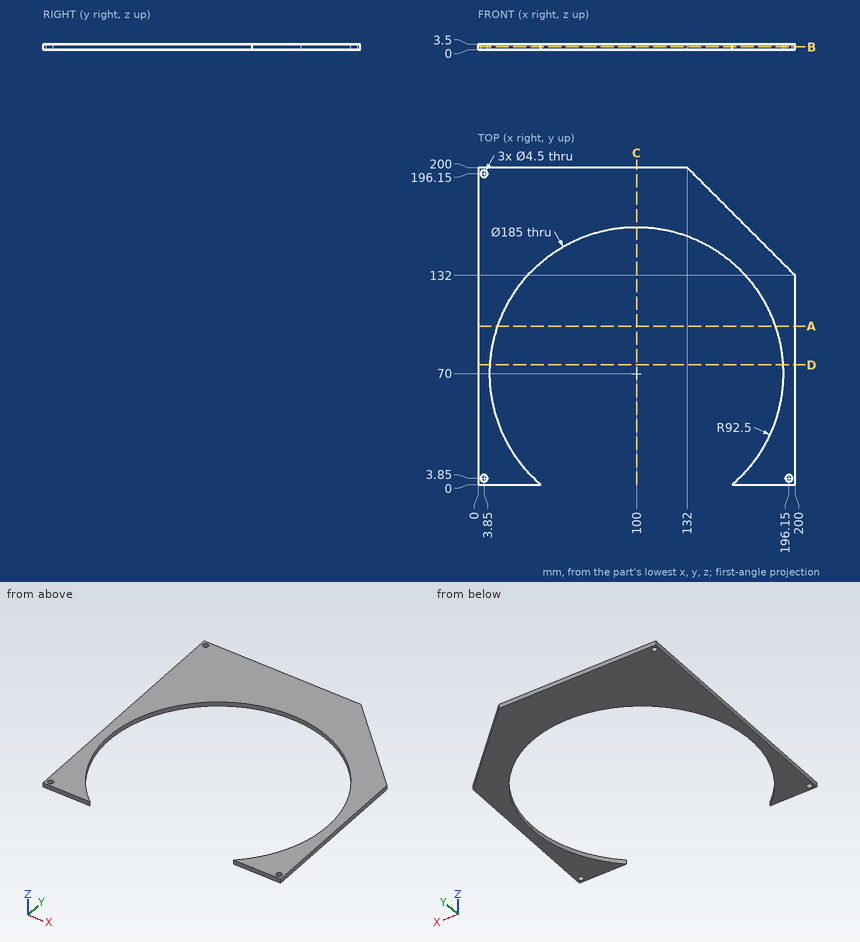
Job drawing, mm, ordinate dimensions from the low corner. One solid piece. Coordinates: 2 decimals unless noted, no trailing zeros. Loops run counter-clockwise (first coordinate to the right, second up) from the corner with the lowest first, then second, coordinate; pieces in that order, holes last. Notation, with made-up numbers: (2.25, 14.25) - (58.25, 14.25) arc R20 cw to (58.25, 39.25) - close; hole circle Ø8 at (-39.5, 29.25). An arc over 180 degrees is marked (long way). Write item = value, one per line. Start each with the question number.
Q1. Flat gauge pins, fed straight in: pin 1 Ø1.5 at (x, z) = (43, 3) entering from -Y; pin 2 Ø4 at (x, y) = (3.85, 3.85) entering from -Z; pin 3 Ø1.5 at (x, z) = (136, 1) entering from -Y. Where does each tip first touch, or does it go through?
Q2. Cut at C-C, the plane x = 100. List the corners of the cut face in (y, z), then the cut area to 3 significant figures.
Q3. Cut at D-D, the plane y = 75.5. List the corners of the cut face in (x, z).
Q4. Drill centre lines: L1, parallel to Y at x = 34, z = 1.85; L2, parallel to Y at x = 175.5, z = 2.6; L3, parallel to X at y = 54.5, z = 0.4. Where is each one in solid material? Low to high.
Q5. Cut at A-A, the plane y = 100. List the corners of the cut face in (x, z).
Q6. Cut at B-B, the plane z = 1.7. List the corners of the cut face in (x, y), then the cut area to 3 significant figures.
Computed:
q1.pin_1 = 142.26
q1.pin_2 = through
q1.pin_3 = 154.89
q2.outline = (162.5, 0) - (200, 0) - (200, 3.5) - (162.5, 3.5) - close
q2.area = 131 mm²
q3.outline = (0, 0) - (7.66, 0) - (7.66, 3.5) - (0, 3.5) - close; (192.34, 0) - (200, 0) - (200, 3.5) - (192.34, 3.5) - close
q4.L1 = 0 to 5.19, 134.81 to 200
q4.L2 = 0 to 16.56, 123.44 to 156.5
q4.L3 = 0 to 8.81, 191.19 to 200
q5.outline = (0, 0) - (12.5, 0) - (12.5, 3.5) - (0, 3.5) - close; (187.5, 0) - (200, 0) - (200, 3.5) - (187.5, 3.5) - close
q6.outline = (0, 0) - (39.53, 0) arc R92.5 cw (long way) to (160.47, 0) - (200, 0) - (200, 132) - (132, 200) - (0, 200) - close; hole circle Ø4.5 at (3.85, 3.85); hole circle Ø4.5 at (3.85, 196.15); hole circle Ø4.5 at (196.15, 3.85)
q6.area = 12,600 mm²
